Job drawing, mm, ordinate dimensions from the low corner. One solid piece. Round coordinates to 2 decimals unless told otherwise and drop trailing zeros. Write each loop counter-clockwise with the first axis right and the second up, starting at its lowest first coordinate (ties: lowest second). Pieces come first, ordered by that corner, then holes. Notation, with made-up numbers: (69.5, 22.5) -> (107.5, 22.5) arc R11 cw to (107.5, 39.5) -> close; hole circle Ø4 at (23, 17.25). An arc over 180 degrees is marked (long way). Use CSV: the item, a comma, the result in double quotes. Start each with the question number.
(1) Saw through at A-A (x = 55). Give the cut face in (y, z) (1 decimal), plus the area to 3 significant figures.
(2) Probe line 1 (Y direction, x = 55, z = 54); line 2 (X direction, y = 56.5, z = 60.5). List the from-to ranges inside material, lowest first. Write a range as [from, to].
(3) Two-plate mould, pull along Z, no slides. Class the marked faces 1, 2 and 3: released by +Z, released by -Z, zero draft, split by the parting line, or undercut.
(4) Saw through at B-B (y = 56). Give the cut face in (x, z) (1 decimal), plus the area to 3 significant figures.
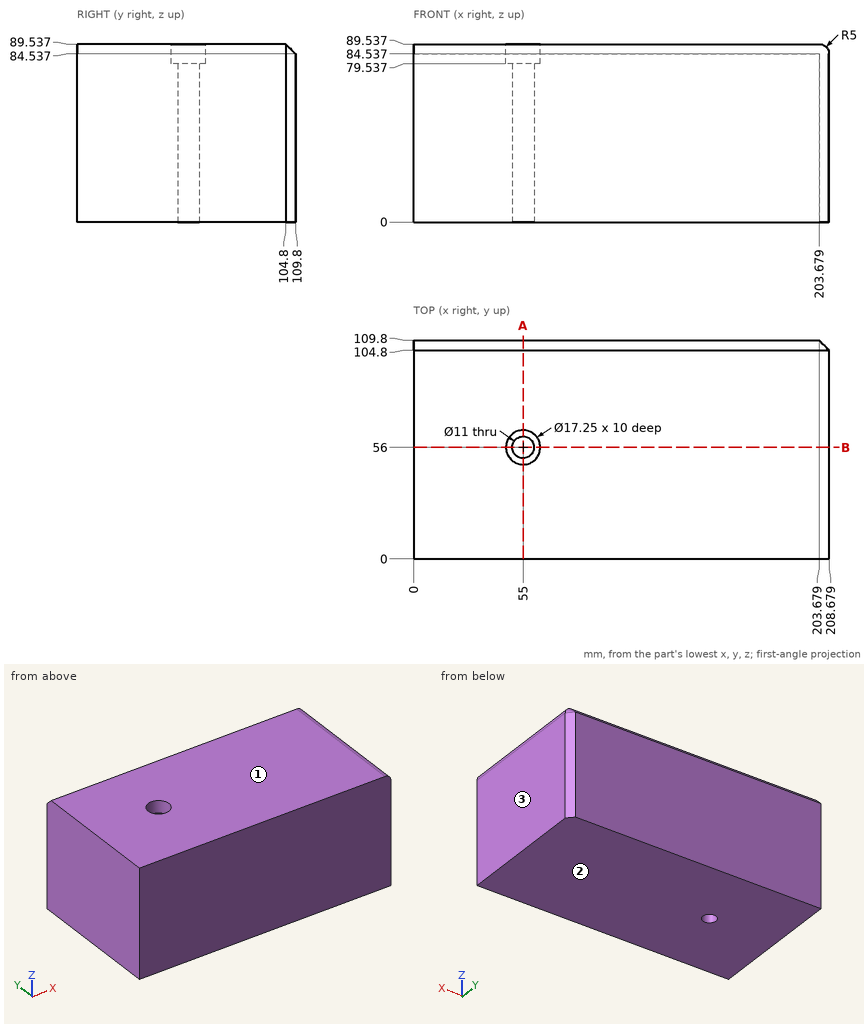
Answers:
1,outline,"(0, 0) -> (50.5, 0) -> (50.5, 79.5) -> (47.4, 79.5) -> (47.4, 89.5) -> (0, 89.5) -> close; (61.5, 0) -> (109.8, 0) -> (109.8, 84.5) -> (104.8, 89.5) -> (64.6, 89.5) -> (64.6, 79.5) -> (61.5, 79.5) -> close"
1,area,"8,770 mm²"
2,line 1,"y = [0, 50.5], [61.5, 109.8]"
2,line 2,"x = [0, 49.52], [60.48, 208.68]"
3,face 1,"released by +Z"
3,face 2,"released by -Z"
3,face 3,"zero draft"
4,outline,"(0, 0) -> (49.5, 0) -> (49.5, 79.5) -> (46.4, 79.5) -> (46.4, 89.5) -> (0, 89.5) -> close; (60.5, 0) -> (208.7, 0) -> (208.7, 84.5) arc R5 ccw to (203.7, 89.5) -> (63.6, 89.5) -> (63.6, 79.5) -> (60.5, 79.5) -> close"
4,area,"17,600 mm²"
